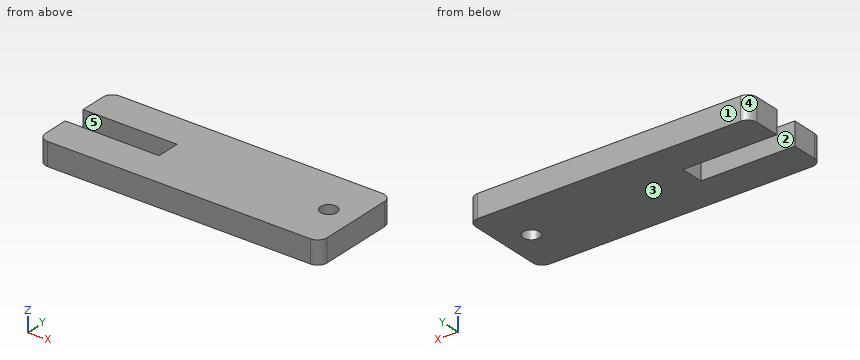
```python
from build123d import *

# Parameters (mm, degrees)
BOSS_EXTRUDE1_DEPTH = 1.5494
FILLET1_R           = 1.27
SKETCH2_R           = 1.1176
CUT_EXTRUDE1_DEPTH  = 27.364465886


with BuildPart() as part:
    # Sketch1 → Boss-Extrude1 (new, symmetric)
    with BuildSketch(Plane.XY):
        Polygon((-12.7, 1.5875), (-12.7, 6.35), (25.4, 6.35), (25.4, -6.35), (-12.7, -6.35), (-12.7, -1.5875), (0, -1.5875), (0, 1.5875), align=None)
    extrude(amount=BOSS_EXTRUDE1_DEPTH, both=True)

    # Fillet1
    fillet1_edges = [part.edges().sort_by_distance(p)[0] for p in [
        (-12.7, 6.35, 0),
        (25.4, 6.35, 0),
        (25.4, -6.35, 0),
        (-12.7, -6.35, 0),
    ]]
    fillet(fillet1_edges, radius=FILLET1_R)

    # Sketch2 → Cut-Extrude1 (cut, through all)
    with BuildSketch(Plane.XY.offset(1.5494)):
        with Locations((21.7424, 0)):
            Circle(SKETCH2_R)
    extrude(amount=-CUT_EXTRUDE1_DEPTH, mode=Mode.SUBTRACT)


solid = part.part
```
Part model, mm, in its own coordinate system. Face numbers are marked on the shaded views. A direction names the side the tool comes from. Give positions to 0.01 mm unless a question says otherwise; leave off trailing zeros. Loops run counter-clockwise (first coordinate to the right, second up) from the corner with the lowest first, then second, coordinate; pieces in that order, holes last. Notation, with made-up numbers: M 48.25,30.5 L 57.25,30.5 A24 ccw 57.25,68.5 Z; hole C 13,45 d5. An arc over 180 degrees is marked long. Return JSON: item names as keys, results as strings.
1) Pull direction Y, two halves, no side cores. Call the marked faces 3, 4 and 5: released by +Y, released by -Y, zero draft, split by the parting line, or undercut.
Calculated:
{"face 3": "zero draft", "face 4": "released by +Y", "face 5": "undercut"}
2) Saw through at A-A, the plane x = -6.5. List the corners of the cut face in (y, z).
Calculated:
{"outline": "M -6.35,-1.55 L -1.59,-1.55 L -1.59,1.55 L -6.35,1.55 Z; M 1.59,-1.55 L 6.35,-1.55 L 6.35,1.55 L 1.59,1.55 Z"}
3) Saw through at B-B, the plane z = -0.2. List the corners of the cut face in (x, y), then the cut area to 3 significant figures.
Calculated:
{"outline": "M -12.7,-5.08 A1.27 ccw -11.43,-6.35 L 24.13,-6.35 A1.27 ccw 25.4,-5.08 L 25.4,5.08 A1.27 ccw 24.13,6.35 L -11.43,6.35 A1.27 ccw -12.7,5.08 L -12.7,1.59 L 0,1.59 L 0,-1.59 L -12.7,-1.59 Z; hole C 21.74,0 d2.24", "area": "438 mm2"}
4) Drill centre lines: line 1 (Y direction, x = -9.5, z = 0.85); line 2 (X direction, y = 5.25, z = -1.1). Where is each one in solid material? Low to high.
Calculated:
{"line 1": "y = -6.35 to -1.59, 1.59 to 6.35", "line 2": "x = -12.69 to 25.39"}
5) 3-axis set-ups, long thin cutter, end or side, ignore diameter. For the marked faces 1 and 2: which of +Z, -Z, +X, -X, +Y, -Y reach the whole face in a straight line?
Calculated:
{"face 1": "+Z, -Z, +X, -X, +Y", "face 2": "+Z, -Z, -X"}
6) Saw through at C-C, the plane y = 0. List the corners of the cut face in (x, z), then the cut area to 3 significant figures.
Calculated:
{"outline": "M 0,-1.55 L 20.62,-1.55 L 20.62,1.55 L 0,1.55 Z; M 22.86,-1.55 L 25.4,-1.55 L 25.4,1.55 L 22.86,1.55 Z", "area": "71.8 mm2"}
